Design review of the part built by this model. Coordinates are the model's own, in mm. A direction names the side the tool comes from. Round coordinates to 2 decimals unless told otherwise and drop trailing zeros. Order: outer loops, then holes, each group sorted by start corner. A loop starts at its lowest first (then second) coordinate and runs counter-clockwise, first axis right, second up. Notation, with made-up numbers: (17.25, 57) - (64.25, 57) arc R18 ccw to (64.25, 86) - close; hole circle Ø3 at (20, 65). An arc over 180 degrees is marked (long way). Use CSV: the item, a comma, the result in double quotes.
Autodesk Inventor part; units mm, degrees
ref_plane "YZ Plane" through (0, 0, 0) normal (1, 0, 0) x (0, 1, 0)
ref_plane "XZ Plane" through (0, 0, 0) normal (0, 1, 0) x (-1, 0, 0)
ref_plane "XY Plane" through (0, 0, 0) normal (0, 0, 1) x (1, 0, 0)
sketch "Sketch1" plane through (0, 0, 0) normal (0, 0, 1) x (1, 0, 0)
  circle A0 centre (0, 0) radius 2.25
  arc A1 (-5.7929, -2.643) -> (-6.5, -3.643) centre (-6.5, -2.893) ccw
  arc A2 (6.5, -3.643) -> (5.7929, -2.643) centre (6.5, -2.893) ccw
  line L0 (-5.7929, -2.643) -> (-4.4568, -2.643)
  line L1 (5.7929, -2.643) -> (4.4568, -2.643)
  arc A3 (3.5185, -1.2971) -> (-3.5185, -1.2971) centre (0, 0) ccw
  arc A4 (-4.4568, -2.643) -> (-3.5185, -1.2971) centre (-4.4568, -1.643) ccw
  arc A5 (3.5185, -1.2971) -> (4.4568, -2.643) centre (4.4568, -1.643) ccw
  line L2 (-0.3, -2.2299) -> (-0.3, -8.643)
  line L3 (0.3, -2.2299) -> (0.3, -3.643)
  arc A6 (-2.7514, -8.9882) -> (-0.3, -8.643) centre (-1.55, -8.643) ccw
  line L4 (-2.7514, -8.9882) -> (-4, -4.643)
  line L5 (-4, -4.643) -> (-1.9, -4.643)
  arc A7 (-1.4986, -8.4691) -> (-1, -8.443) centre (-1.25, -8.443) ccw
  line L6 (-1.9, -4.643) -> (-1.4986, -8.4691)
  line L7 (-1, -3.643) -> (-1, -8.443)
  line L8 (-12.8733, -3.643) -> (-1, -3.643)
  line L9 (1, -3.643) -> (16.2885, -3.643)
  line L10 (0, 6.5107) -> (0, -12.8141)
  line L11 (0.3, -2.2299) -> (0.3, -8.643)
  arc A8 (0.3, -8.643) -> (2.7514, -8.9882) centre (1.55, -8.643) ccw
  line L12 (2.7514, -8.9882) -> (4, -4.643)
  line L13 (4, -4.643) -> (1.9, -4.643)
  arc A9 (1, -8.443) -> (1.4986, -8.4691) centre (1.25, -8.443) ccw
  line L14 (1.9, -4.643) -> (1.4986, -8.4691)
  line L15 (1, -3.643) -> (1, -8.443)
  dimension "d0" = 4.5
  dimension "d5" = 1.5
  dimension "d6" = 1.5
  dimension "d7" = 6.5
  dimension "d8" = 6.5
  dimension "d9" = 3.75
  dimension "d10" = 1
  dimension "d11" = 0.6
  dimension "d12" = 0.3
  dimension "d13" = 0.5
  dimension "d14" = 2.5
  dimension "d15" = 4
  dimension "d17" = 2.1
  dimension "d18" = 0.2
  dimension "d19" = 0.7
  dimension "d21" = 3.643
  dimension "d22" = 1
  dimension "d23" = 1
  dimension "d24" = 5
  dimension "d25" = 1
extrude "Extrusion1" add sketch "Sketch1" along normal mid plane 10 contours A0 L10 A3 A5 L1 A2 L9 L15 A9 L14 L13 L12 A8 L11 L3 | A0 L2 A6 L4 L5 L6 A7 L7 L8 A1 L0 A4 A3 L10
sketch "Sketch2" plane through (1, -3.643, 5) normal (0, -1, 0) x (1, 0, 0)
  circle A0 centre (-1, -5) radius 10
  circle A1 centre (-1, -5) radius 5
  dimension "d28" = 10
  dimension "d29" = 5
extrude "Extrusion2" cut sketch "Sketch2" along normal through all
sketch "Sketch3" plane through (0, 0, 0) normal (1, 0, 0) x (0, 1, 0)
  line L0 (-3.643, 5) -> (-3.643, 4.991)
  line L1 (-3.643, -5) -> (-3.643, 5)
  line L2 (-3.643, -4.991) -> (-3.643, -5)
  line L3 (-3.643, -4.899) -> (-3.643, -4.991)
  line L4 (-3.643, -4.899) -> (-3.643, 4.899)
  line L5 (-3.643, 4.991) -> (-3.643, 4.899)
  line L6 (-3.643, 5) -> (-3.643, 4.5)
  line L7 (-11.643, 3.8876) -> (-11.643, 6)
  line L8 (-11.643, 6) -> (-3.643, 6)
  line L9 (-3.643, 6) -> (-3.643, 5)
  line L10 (-3.643, 4.5) -> (-4.643, 4.5)
  line L11 (-4.643, 4.5) -> (-11.643, 3.8876)
  line L12 (-13.9716, 0) -> (2.3286, 0)
  line L13 (-3.643, -5) -> (-3.643, -4.991)
  line L14 (-3.643, -4.991) -> (-3.643, -4.899)
  line L15 (-3.643, -5) -> (-3.643, -4.5)
  line L16 (-11.643, -3.8876) -> (-11.643, -6)
  line L17 (-11.643, -6) -> (-3.643, -6)
  line L18 (-3.643, -6) -> (-3.643, -5)
  line L19 (-3.643, -4.5) -> (-4.643, -4.5)
  line L20 (-4.643, -4.5) -> (-11.643, -3.8876)
  point P0 (0, 0)
  dimension "d32" = 1
  dimension "d33" = 5
  dimension "d34" = 0.5
  dimension "d35" = 1
  dimension "d36" = 8
extrude "Extrusion3" cut sketch "Sketch3" along normal through all both and the other way through all
equation "\"d6\" = d5"
equation "\"d4\" = d3"
properties part number "202-15" material "ABS Plastic"
1) We need section D-D (z = -2.25). Give the boundary of the cut face in (x, y).
Data:
outline,"(-6.5, -3.64) - (-1, -3.64) - (-1, -8.44) arc R0.25 cw to (-1.5, -8.47) - (-1.9, -4.64) - (-4, -4.64) - (-2.75, -8.99) arc R1.25 ccw to (-0.3, -8.64) - (-0.3, -2.23) arc R2.25 cw (long way) to (0.3, -2.23) - (0.3, -8.64) arc R1.25 ccw to (2.75, -8.99) - (4, -4.64) - (1.9, -4.64) - (1.5, -8.47) arc R0.25 cw to (1, -8.44) - (1, -3.64) - (6.5, -3.64) arc R0.75 ccw (long way) to (5.79, -2.64) - (4.46, -2.64) arc R1 cw to (3.52, -1.3) arc R3.75 ccw (long way) to (-3.52, -1.3) arc R1 cw to (-4.46, -2.64) - (-5.79, -2.64) arc R0.75 ccw (long way) to start"
2) The part is to be moulded in two halves that separate along X. For faces 1 (the face through (1.815, -7.231, -4.274)), 2 (the face through (3, -6, 4)), 3 (the face through (-1.351, -9.877, -0.058)), say which applies: +X half, -X half, draft (parallel to the pull), parting line (faces both ways), or undercut.
Data:
face 1,"draft"
face 2,"+X half"
face 3,"undercut"
3) We need section C-C (y = -5.25). Give the boundary of the cut face in (x, z).
Data:
outline,"(-3.83, -3.22) arc R5 ccw to (-2.29, -4.45) - (-1.84, -4.45) - (-1.84, 4.45) - (-2.29, 4.45) arc R5 ccw to (-3.83, 3.22) - close; (-1, -4.45) - (-0.3, -4.45) - (-0.3, 4.45) - (-1, 4.45) - close; (0.3, -4.45) - (1, -4.45) - (1, 4.45) - (0.3, 4.45) - close; (1.84, -4.45) - (2.29, -4.45) arc R5 ccw to (3.83, -3.22) - (3.83, 3.22) arc R5 ccw to (2.29, 4.45) - (1.84, 4.45) - close"
4) For faces 4 (the face through (-3, -6, -4)), 5 (the face through (0.3, -5, 0)), 6 (the face through (-3, -4.643, 0)), list the 3-axis set-ups (+Z, -Z, +X, -X, +Y, -Y) from which the entire face can be reached by the end or side of a thin tool; tool diameter is ignored.
Data:
face 4,"-Z, -X, -Y"
face 5,"+Z, -Z, -Y"
face 6,"+Z, -Z, -X"
5) We need section B-B (x = 0.75). Give the boundary of the cut face in (y, z), then the cut area to 3 significant figures.
Data:
outline,"(-9.6, -4.07) - (-4.64, -4.5) - (-3.64, -4.5) - (-3.64, -5) - (-2.12, -5) - (-2.12, 5) - (-3.64, 5) - (-3.64, 4.5) - (-4.64, 4.5) - (-9.6, 4.07) - close; (2.12, -5) - (3.67, -5) - (3.67, 5) - (2.12, 5) - close"
area,"82.2 mm2"
6) To check wall thickness, follow L1, parallel to X at y = 0, z = -2; L2, parallel to X at y = -4, z = -3.5; L3, parallel to Y at x = 1.25, z = 2.5. State the ranges of each line that lie inside material, in increasing order. Write a range as from..to.
Data:
L1,"x = -3.75..-2.25, 2.25..3.75"
L2,"x = -1..-0.3, 0.3..1"
L3,"y = -9.86..-8.69, -3.64..-1.87, 1.87..3.54"
7) We need section A-A (y = 0). Give the boundary of the cut face in (x, z).
Data:
outline,"(-3.75, -5) - (-2.25, -5) - (-2.25, 5) - (-3.75, 5) - close; (2.25, -5) - (3.75, -5) - (3.75, 5) - (2.25, 5) - close"
8) Insertion check: pin 1 Ø0.6 at (x, y) = (0.5, -4) entering from +Z; pin 2 Ø4 at (y, z) = (-7, 2) entering from -X; pin 3 Ø3 at (x, y) = (0.5, -7.5) entering from -Z. Each pin has a flat end and moves straight along its axis. Give the tip position at first contact, or say it passes through.
Data:
pin 1,"stops at z = 4.5"
pin 2,"stops at x = -3.9"
pin 3,"stops at z = -4.38"
